Answer from the drawing. Dimensions are ordinates in mm from the lowest x, y and z of the part. A direction names the side the tool comes from. Round coordinates to 2 decimals unless told otherwise and drop trailing zeros. Write each loop counter-clockwise with the first axis right and the second up, starting at its lowest first coordinate (ties: lowest second). Pieces come first, ordered by that corner, then holes. Notation, with made-up numbers: (47, 3) -> (102, 3) arc R16 cw to (102, 24) -> close; hole circle Ø8 at (-21, 42.25). An arc over 180 degrees is marked (long way). Return JSON: item names as keys, results as strings. Group by question number.
(1) A cutting plane is placed at C-C on z = 6. Give the vertices of the cut face in (x, y), then the cut area to 3 significant figures.
(2) Given pin 1 (0.9 mm diameter, centred on x = 6, z = 1.5, fed in from -Y); pin 2 (1 mm diameter, centred on y = 1.5, z = 13, fed in from -X); pin 3 (1 mm diameter, centred on y = 5.5, z = 8, fed in from -X), each flat-ended and moving along its own axis, determine where each tip first touches the part or whether it passes through.
(3) The mould has two halves that part along Z. Classify the marked faces 1, 2 and 3: released by +Z, released by -Z, zero draft, split by the parting line, or undercut.
(4) A cutting plane is placed at A-A on x = 10. Give the vertices of the cut face in (y, z), then the cut area to 3 significant figures.
(5) Straight lines are drawn through the part: line 1 (Z direction, x = 4.5, y = 5); line 2 (X direction, y = 4.5, z = 21.5); line 3 (X direction, y = 2.75, z = 11.5). For each, find the intervals that lie inside material, in ascending order.
(6) For the marked faces 4, 5 and 6, determine the directions among +Z, -Z, +X, -X, +Y, -Y from which every point of the face is accessible in a straight line to the end or side of a thin tool.
(7) A cutting plane is placed at B-B on x = 15. Give the vertices of the cut face in (y, z), then the cut area to 3 significant figures.
(8) A cutting plane is placed at D-D on y = 1.5. Give the vertices of the cut face in (x, z).
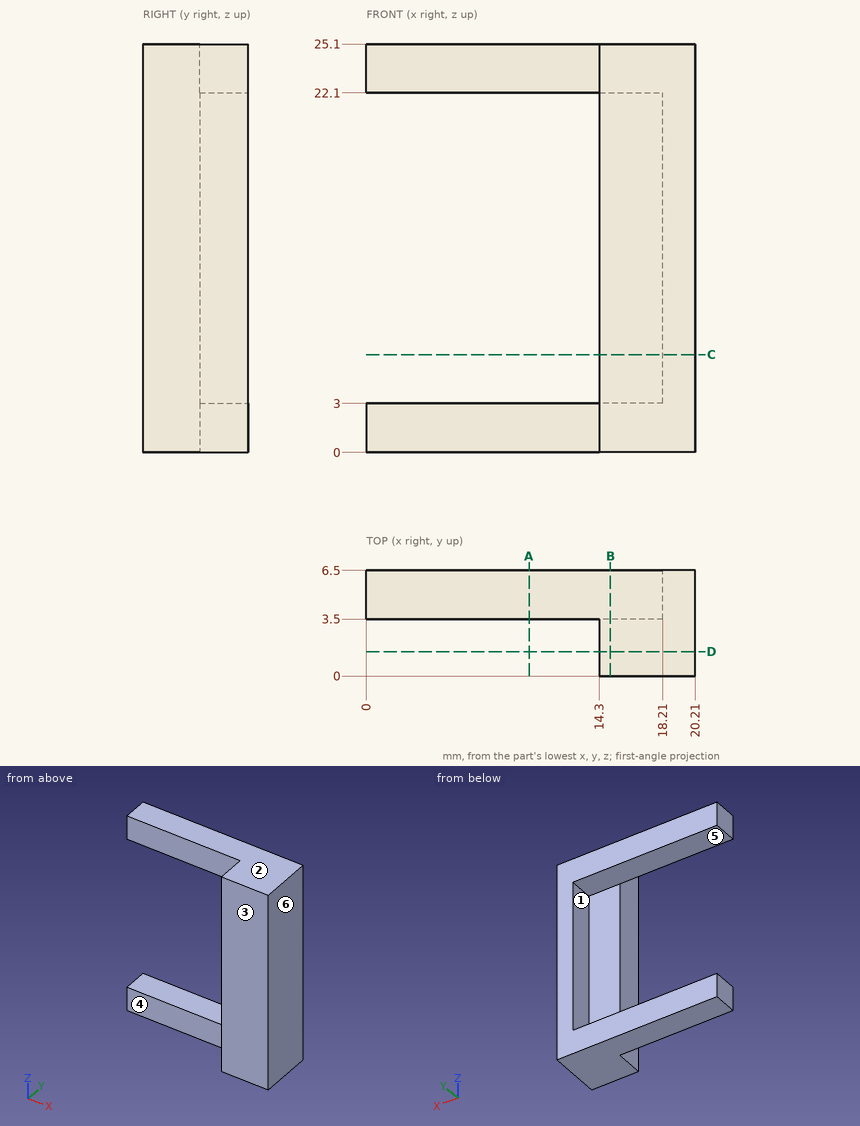
Checks:
{
 "1": {"outline": "(14.3, 0) -> (20.21, 0) -> (20.21, 6.5) -> (18.21, 6.5) -> (18.21, 3.5) -> (14.3, 3.5) -> close", "area": "26.7 mm^2"},
 "2": {"pin 1": "stops at y = 3.5", "pin 2": "stops at x = 14.3", "pin 3": "stops at x = 18.21"},
 "3": {"face 1": "undercut", "face 2": "released by +Z", "face 3": "zero draft"},
 "4": {"outline": "(3.5, 0) -> (6.5, 0) -> (6.5, 3) -> (3.5, 3) -> close; (3.5, 22.1) -> (6.5, 22.1) -> (6.5, 25.1) -> (3.5, 25.1) -> close", "area": "18.0 mm^2"},
 "5": {"line 1": "z = 0 to 3, 22.1 to 25.1", "line 2": "x = 18.21 to 20.21", "line 3": "x = 14.3 to 20.21"},
 "6": {"face 4": "+Z, -Z, -X, -Y", "face 5": "-X, +Y", "face 6": "+Z, -Z, +X, +Y, -Y"},
 "7": {"outline": "(0, 0) -> (6.5, 0) -> (6.5, 3) -> (3.5, 3) -> (3.5, 22.1) -> (6.5, 22.1) -> (6.5, 25.1) -> (0, 25.1) -> close", "area": "106 mm^2"},
 "8": {"outline": "(14.3, 0) -> (20.21, 0) -> (20.21, 25.1) -> (14.3, 25.1) -> close"}
}
